from build123d import *

# Parameters (mm, degrees)
SKETCH1_W            = 53.5
SKETCH1_H            = 30
BOSS_EXTRUDE1_DEPTH  = 2.3114
SKETCH2_W            = 2.3114
SKETCH2_H            = 30
BOSS_EXTRUDE2_DEPTH  = 16
BOSS_EXTRUDE3_DEPTH  = 2.3114
FILLET1_R            = 1
FILLET2_START        = -16
FILLET2_DEPTH        = 32
BOSS_EXTRUDE5_DEPTH  = 1
MIRROR3_COPY_1_DEPTH = 1


with BuildPart() as part:
    # Sketch1 → Boss-Extrude1 (new body)
    with BuildSketch(Plane.XY):
        Rectangle(SKETCH1_W, SKETCH1_H)
    extrude(amount=BOSS_EXTRUDE1_DEPTH)

    # Sketch2 → Boss-Extrude2 (add)
    with BuildSketch(Plane.XY.offset(2.3114)):
        with Locations((-25.5943, 0)):
            Rectangle(SKETCH2_W, SKETCH2_H)
    extrude(amount=BOSS_EXTRUDE2_DEPTH)

    # Sketch3 → Boss-Extrude3 (add)
    with BuildSketch(Plane.XZ.offset(15)):
        Polygon((-24.4386, 18.3114), (2.5614, 2.3114), (-24.4386, 2.3114), align=None)
    boss_extrude3 = extrude(amount=-BOSS_EXTRUDE3_DEPTH)

    # Mirror1: Boss-Extrude3 across plane
    add(boss_extrude3.mirror(Plane.ZX))

    # Fillet1
    fillet1_edges = [part.edges().sort_by_distance(p)[0] for p in [
        (26.75, 15, 1.1557),
        (26.75, -15, 1.1557),
        (-26.75, 15, 9.1557),
        (-26.75, -15, 9.1557),
    ]]
    fillet(fillet1_edges, radius=FILLET1_R)

    # Fillet2: read off the stored shape, not the designer's step
    # Fillet2 outline → Fillet2 (cut)
    with BuildSketch(Plane(origin=(0, 0, 0), x_dir=(1, 0, 0), z_dir=(0, 1, 0)).offset(FILLET2_START)):
        with BuildLine():
            Line((-24.4386, -18.3114), (-23.259809815, -17.612857668))
            ThreePointArc((-23.259809815, -17.612857668), (-24.487324196, -18.133603249), (-25.808821767, -18.3114))
            Line((-25.808821767, -18.3114), (-24.4386, -18.3114))
        make_face()
    extrude(amount=FILLET2_DEPTH, mode=Mode.SUBTRACT)

    # Sketch7 → Boss-Extrude5 (add)
    with BuildSketch(Plane(origin=(0, 0, 0), x_dir=(-1, 0, 0), z_dir=(0, 0, -1))):
        with BuildLine():
            Line((-25.75, 15), (-21.75, 15))
            Line((-21.75, 15), (-21.75, 14.5))
            Line((-21.75, 14.5), (-25.75, 14.5))
            ThreePointArc((-25.75, 14.5), (-26.103553391, 14.353553391), (-26.25, 14))
            Line((-26.25, 14), (-26.25, 10))
            Line((-26.25, 10), (-26.75, 10))
            Line((-26.75, 10), (-26.75, 14))
            ThreePointArc((-26.75, 14), (-26.457106781, 14.707106781), (-25.75, 15))
        make_face()
    boss_extrude5 = extrude(amount=BOSS_EXTRUDE5_DEPTH)

    # Mirror2: Boss-Extrude5 across plane
    add(boss_extrude5.mirror(Plane.ZX))

    # Mirror3: Boss-Extrude5 across plane
    add(boss_extrude5.mirror(Plane(origin=(0, 0, 0), x_dir=(0, 0, 1), z_dir=(1, 0, 0))))

    # Mirror3 copy 1 sketch → Mirror3 copy 1 (add)
    with BuildSketch(Plane(origin=(0, 0, 0), x_dir=(1, 0, 0), z_dir=(0, 0, -1))):
        with BuildLine():
            Line((-25.75, 15), (-21.75, 15))
            Line((-21.75, 15), (-21.75, 14.5))
            Line((-21.75, 14.5), (-25.75, 14.5))
            ThreePointArc((-25.75, 14.5), (-26.103553391, 14.353553391), (-26.25, 14))
            Line((-26.25, 14), (-26.25, 10))
            Line((-26.25, 10), (-26.75, 10))
            Line((-26.75, 10), (-26.75, 14))
            ThreePointArc((-26.75, 14), (-26.457106781, 14.707106781), (-25.75, 15))
        make_face()
    extrude(amount=MIRROR3_COPY_1_DEPTH)


solid = part.part
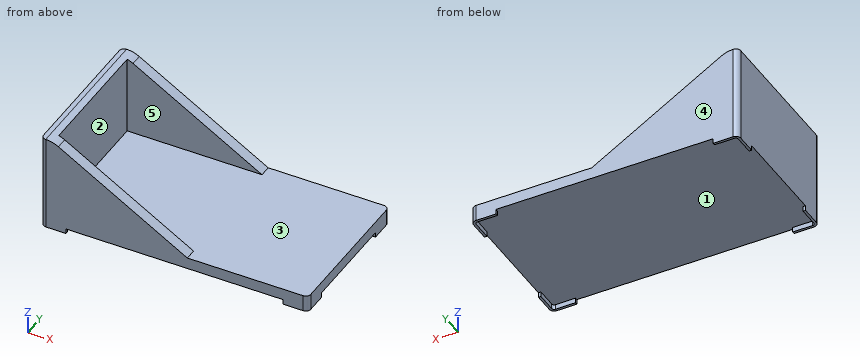
Build history of the part. All positions in model axes, mm. Face numbers are marked on the shaded views. A direction names the side the tool comes from. Round coordinates to 2 decimals unless told otherwise and drop trailing zeros. Loops run counter-clockwise (first coordinate to the right, second up) from the corner with the lowest first, then second, coordinate; pieces in that order, holes last. Notation, with made-up numbers: (53.5, -34) -> (61.5, -34) arc R11 cw to (61.5, -29) -> close; hole circle Ø10 at (-18.5, 77.5). An arc over 180 degrees is marked (long way). Answer in a Markdown table with one row per item.
Item 1: Saw through at B-B (y = 7). Write the cut outline in (x, z), and give its area (3 significant figures).
Answers below:
| item | result |
|---|---|
| outline | (-26.75, 0) -> (26.75, 0) -> (26.75, 2.31) -> (-24.44, 2.31) -> (-24.44, 18.12) arc R5 ccw to (-25.81, 18.31) -> (-26.75, 18.31) -> close |
| area | 161 mm² |
Item 2: Saw through at A-A (x = -8). Write the cut outline in (y, z).
Answers below:
| item | result |
|---|---|
| outline | (-15, 0) -> (15, 0) -> (15, 8.57) -> (12.69, 8.57) -> (12.69, 2.31) -> (-12.69, 2.31) -> (-12.69, 8.57) -> (-15, 8.57) -> close |
Item 3: Drill centre lines: L1, parallel to Y at x = -7, z = 3.5; L2, parallel to Z at x = -19, y = -7.5; L3, parallel to X at y = 10.5, z = 10. Where is each one in solid material? Low to high. Write a range as [from, to].
Answers below:
| item | result |
|---|---|
| L1 | y = [-15, -12.69], [12.69, 15] |
| L2 | z = [0, 2.31] |
| L3 | x = [-26.75, -24.44] |
Item 4: Which spindle directions (+Z, -Z, +X, -X, +Y, -Y) get a long thin tool onto all of the face, cutting with end or side? Do the marked faces 4 and 5. Say none if no direction does.
Answers below:
| item | result |
|---|---|
| face 4 | +Z, -Z, +X, -X, +Y |
| face 5 | +Z, +X |
Item 5: Pin check, flat tips, straight feed: pin 1 (3 mm diameter, centred on x = -13, y = -9.5, fed in from -Z); pin 2 (1 mm diameter, centred on x = 17, y = 10.5, fed in from +Z); pin 3 (0.6 mm diameter, centred on y = 14.5, z = -0.5, fed in from -X); pin 4 (6 mm diameter, centred on x = 10.5, z = 6, fed in from +Y). Stop position of each tip, or through.
Answers below:
| item | result |
|---|---|
| pin 1 | stops at z = 0 |
| pin 2 | stops at z = 2.31 |
| pin 3 | stops at x = -26.73 |
| pin 4 | passes through |
Item 6: Saw through at C-C (z = 15.75). Write the cut outline in (x, y), and give its area (3 significant figures).
Answers below:
| item | result |
|---|---|
| outline | (-26.75, -14) arc R1 ccw to (-25.75, -15) -> (-20.12, -15) -> (-20.12, -12.69) -> (-24.44, -12.69) -> (-24.44, 12.69) -> (-20.12, 12.69) -> (-20.12, 15) -> (-25.75, 15) arc R1 ccw to (-26.75, 14) -> close |
| area | 88.9 mm² |
Item 7: Saw through at D-D (x = 1). Write the cut outline in (y, z), and give its area (3 significant figures).
Answers below:
| item | result |
|---|---|
| outline | (-15, 0) -> (15, 0) -> (15, 3.24) -> (12.69, 3.24) -> (12.69, 2.31) -> (-12.69, 2.31) -> (-12.69, 3.24) -> (-15, 3.24) -> close |
| area | 73.6 mm² |
Item 8: Mould opens along X. For the marked faces 1, 2 and 3 say: +X half, -X half, draft (parallel to the pull), parting line (faces both ways), or undercut.
Answers below:
| item | result |
|---|---|
| face 1 | undercut |
| face 2 | +X half |
| face 3 | draft |
